The listing builds one solid part. Answer for the finished solid, in the listing's coordinates (mm). Face numbers are marked on the shaded views. Give positions to 0.01 mm unless a question says otherwise; leave off trailing zeros. Loops run counter-clockwise (first coordinate to the right, second up) from the corner with the lowest first, then second, coordinate; pieces in that order, holes last. Notation, with made-up numbers: (82.25, 64) - (120.25, 64) arc R20 ccw to (120.25, 99) - close; hole circle Ø10 at (80, 77.25). An arc over 180 degrees is marked (long way). Answer as CSV lines item,"result". Start each with the question number.
1) A flat-ended cylindrical pin translates along its axis: pin 1 (1 mm diameter, centred on x = -1, z = 0.5, fed in from -Y). Find the tip coordinate at first contact, or state that the pin passes through.
2) For a pull along Y with two mould halves and no side action, classify the marked faces 1 and 2 as pulls with the +Y half, pulls with the -Y half, needs draft (parallel to the pull), parting line crosses it, or undercut.
3) A cutting plane is placed at A-A (y = 0). Determine the outline of the cut face in (x, z).
4) Find the intervals of material crossed by line 1 along Z through (x, y) = (-0.35, -1.1); line 2 along Z through (x, y) = (-1.3, 0.15); line 3 along X through (y, z) = (-0.2, -4), in increasing order.
5) A cutting plane is placed at C-C (z = 4.25). Determine the outline of the cut face in (x, y).
```python
from build123d import *

# Parameters (mm, degrees)
SKETCH1_R           = 1.4986
BOSS_EXTRUDE1_DEPTH = 5.55625
SKETCH2_W           = 0.54
SKETCH2_H           = 0.5461
CHAMFER1_SIZE       = 0.254


with BuildPart() as part:
    # Sketch1 → Boss-Extrude1 (new body, symmetric)
    with BuildSketch(Plane.XY):
        Circle(SKETCH1_R)
    extrude(amount=BOSS_EXTRUDE1_DEPTH, both=True)

    # Sketch2 → Cut-Revolve1 (revolve, cut)
    with BuildSketch(Plane(origin=(0, 0, 0), x_dir=(0, 0, -1), z_dir=(1, 0, 0))):
        with Locations((-4.77825, -1.22555)):
            Rectangle(SKETCH2_W, SKETCH2_H)
        with Locations((4.77825, -1.22555)):
            Rectangle(SKETCH2_W, SKETCH2_H)
    revolve(axis=Axis((0, 0, 8.828032455), (0, 0, -1)), mode=Mode.SUBTRACT)

    # Chamfer1
    chamfer1_edges = [part.edges().sort_by_distance(p)[0] for p in [
        (-1.4986, 0, -5.55625),
        (-1.4986, 0, 5.55625),
    ]]
    chamfer(chamfer1_edges, length=CHAMFER1_SIZE)


solid = part.part
```
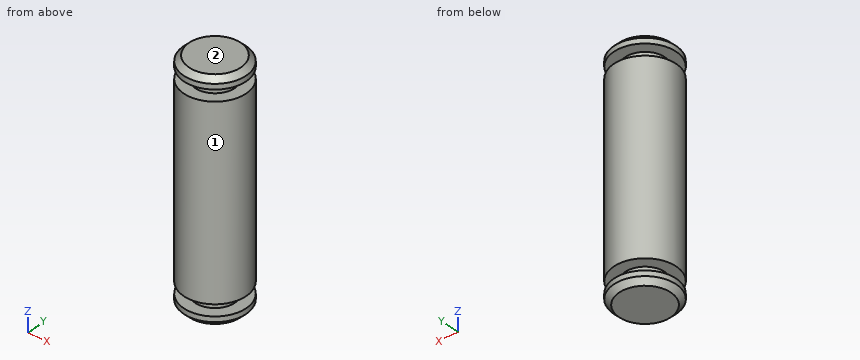
Ans:
1,pin 1,"y = -1.41"
2,face 1,"parting line crosses it"
2,face 2,"needs draft"
3,outline,"(-1.5, -5.3) - (-1.24, -5.56) - (1.24, -5.56) - (1.5, -5.3) - (1.5, -5.05) - (0.95, -5.05) - (0.95, -4.51) - (1.5, -4.51) - (1.5, 4.51) - (0.95, 4.51) - (0.95, 5.05) - (1.5, 5.05) - (1.5, 5.3) - (1.24, 5.56) - (-1.24, 5.56) - (-1.5, 5.3) - (-1.5, 5.05) - (-0.95, 5.05) - (-0.95, 4.51) - (-1.5, 4.51) - (-1.5, -4.51) - (-0.95, -4.51) - (-0.95, -5.05) - (-1.5, -5.05) - close"
4,line 1,"-5.56 to -5.05, -4.51 to 4.51, 5.05 to 5.56"
4,line 2,"-5.49 to -5.05, -4.51 to 4.51, 5.05 to 5.49"
4,line 3,"-1.49 to 1.49"
5,outline,"circle Ø3 at (0, 0)"
